```python
from build123d import *

# Parameters (mm, degrees)
SKETCH1_W                                        = 203.2
SKETCH1_H                                        = 203.2
BOSS_EXTRUDE1_DEPTH                              = 38.1
CBORE_FOR_1_2_SOCKET_HEAD_CAP_SCREW1_D           = 13.09624
CBORE_FOR_1_2_SOCKET_HEAD_CAP_SCREW1_CBORE_D     = 20.6375
CBORE_FOR_1_2_SOCKET_HEAD_CAP_SCREW1_CBORE_DEPTH = 19.05


with BuildPart() as part:
    # Sketch1 → Boss-Extrude1 (new body)
    with BuildSketch(Plane.XY):
        Rectangle(SKETCH1_W, SKETCH1_H)
    extrude(amount=BOSS_EXTRUDE1_DEPTH)

    # CBORE for 1/2 Socket Head Cap Screw1 (through all)
    with Locations(Plane.XY.offset(38.1)):
        with Locations((44.45, -44.45), (-44.45, -44.45), (-44.45, 44.45), (44.45, 44.45)):
            CounterBoreHole(CBORE_FOR_1_2_SOCKET_HEAD_CAP_SCREW1_D / 2, CBORE_FOR_1_2_SOCKET_HEAD_CAP_SCREW1_CBORE_D / 2, CBORE_FOR_1_2_SOCKET_HEAD_CAP_SCREW1_CBORE_DEPTH)


solid = part.part
```
The listing builds one solid part. Answer for the finished solid, in the listing's coordinates (mm). A direction names the side the tool comes from. Round coordinates to 2 decimals unless told otherwise and drop trailing zeros. Loops run counter-clockwise (first coordinate to the right, second up) from the corner with the lowest first, then second, coordinate; pieces in that order, holes last.
1) A cutting plane is placed at C-C on z = 23.5. Determine the outline of the cut face in (x, y), plus the area to 3 significant figures.
Outcome:
outline: (-101.6, -101.6) - (101.6, -101.6) - (101.6, 101.6) - (-101.6, 101.6) - close; hole circle Ø20.64 at (-44.45, -44.45); hole circle Ø20.64 at (-44.45, 44.45); hole circle Ø20.64 at (44.45, -44.45); hole circle Ø20.64 at (44.45, 44.45)
area: 40,000 mm2
2) Given P1, Ø10.5, axis at x = 42, y = -47, coming from the +Z side; P2, Ø6, axis at x = -43, y = 42.5, coming from the +Z side, each flat-ended and moving along its own axis, determine where each tip first touches the part or whether it passes through.
Outcome:
P1: stops at z = 19.05
P2: passes through
3) For a pull along X with two mould halves and no side action, classify faces 3 (the face through (-1, 101.6, 19)), 4 (the face through (49.276, 48.876, 9.392)), 5 (the face through (-101.6, -1, 19)), 6 (the face through (101.6, -1, 19)) as released by +X, released by -X, zero draft, split by the parting line, or undercut.
Outcome:
face 3: zero draft
face 4: undercut
face 5: released by -X
face 6: released by +X
4) A cutting plane is placed at A-A on y = -44.45. Determine the outline of the cut face in (x, z), plus the area to 3 significant figures.
Outcome:
outline: (-101.6, 0) - (-51, 0) - (-51, 19.05) - (-54.77, 19.05) - (-54.77, 38.1) - (-101.6, 38.1) - close; (-37.9, 0) - (37.9, 0) - (37.9, 19.05) - (34.13, 19.05) - (34.13, 38.1) - (-34.13, 38.1) - (-34.13, 19.05) - (-37.9, 19.05) - close; (51, 0) - (101.6, 0) - (101.6, 38.1) - (54.77, 38.1) - (54.77, 19.05) - (51, 19.05) - close
area: 6,460 mm2
5) Consider line 1 (Y direction, x = 44.45, z = 25.5); line 2 (X direction, y = -44, z = 32); line 3 (X direction, y = -42, z = 32). Determine where each line is inside the solid, lowest interval first.
Outcome:
line 1: y = -101.6 to -54.77, -34.13 to 34.13, 54.77 to 101.6
line 2: x = -101.6 to -54.76, -34.14 to 34.14, 54.76 to 101.6
line 3: x = -101.6 to -54.47, -34.43 to 34.43, 54.47 to 101.6
6) For faces 1 (the face through (-43.598, 50.942, 9.392)), 2 (the face through (44.3, 37.7, 19.05)), determine the directions among +Z, -Z, +X, -X, +Y, -Y from which every point of the face is accessible in a straight line to the end or side of a thin tool.
Outcome:
face 1: +Z, -Z
face 2: +Z
